Build history of the part. All positions in model axes, mm. A direction names the side the tool comes from. Round coordinates to 2 decimals unless told otherwise and drop trailing zeros. Order: outer loops, then holes, each group sorted by start corner. A loop starts at its lowest first (then second) coordinate and runs counter-clockwise, first axis right, second up. Notation, with made-up numbers: M 23,31 L 34,31 A17 ccw 34,35 Z; hole C -22,18.25 d3. An arc over 180 degrees is marked long. One line per question, with ' | ' between items. Start each with the question number.
from build123d import *

# Parameters (mm, degrees)
SM_BASE_FLANGE_1_DEPTH = 20
HOLE_WIZARD_M51_D      = 5.2
HOLE_WIZARD_M51_DEPTH  = 10
HOLE_WIZARD_M51_TIP    = 1.562237609


# Sheet-metal steps are written as plain solids
with BuildPart() as part:
    # Sketch 1 → Базовая кромка1 (new body)
    with BuildSketch(Plane(origin=(0, 0, 0), x_dir=(0, 0, -1), z_dir=(1, 0, 0))):
        with BuildLine():
            Line((0, 0), (0, 20))
            ThreePointArc((0, 20), (2.928932188, 27.071067812), (10, 30))
            Line((10, 30), (48.1, 30))
            ThreePointArc((48.1, 30), (55.171067812, 27.071067812), (58.1, 20))
            Line((58.1, 20), (58.1, 0))
            Line((58.1, 0), (68.1, 0))
            Line((68.1, 0), (68.1, 20))
            ThreePointArc((68.1, 20), (62.242135624, 34.142135624), (48.1, 40))
            Line((48.1, 40), (10, 40))
            ThreePointArc((10, 40), (-4.142135624, 34.142135624), (-10, 20))
            Line((-10, 20), (-10, 0))
            Line((-10, 0), (0, 0))
        make_face()
    extrude(amount=SM_BASE_FLANGE_1_DEPTH)

    # Сверло под метчик  спиральное M51
    with Locations(Plane(origin=(0, 0, 0), x_dir=(-1, 0, 0), z_dir=(0, -1, 0))):
        with Locations((-10, 63.1), (-10, -5)):
            Hole(HOLE_WIZARD_M51_D / 2, depth=HOLE_WIZARD_M51_DEPTH)
            with Locations((0, 0, -(HOLE_WIZARD_M51_DEPTH + HOLE_WIZARD_M51_TIP / 2))):  # 118° drill point
                Cone(0, HOLE_WIZARD_M51_D / 2, HOLE_WIZARD_M51_TIP, mode=Mode.SUBTRACT)


solid = part.part
Item 1: Tool access for faces 1 (the face through (9.86, 33.986, -62.397)), 2 (the face through (10, 30, -29)), 3 (the face through (9.662, 5.07, -65.678)): list every direction of +Z, -Z, +X, -X, +Y, -Y with a clear straight run to the whole face (end or side of a thin tool).
Item 2: Flat gauge pins, fed straight in: pin 1 (10 mm diameter, centred on x = 3, y = 30.5, fed in from +Z); pin 2 (4.5 mm diameter, centred on x = 10, z = 5, fed in from +Y); pin 3 (3 mm diameter, centred on x = 6, y = 34, fed in from -Z). Where does each tip first touch, or does it go through?
Item 3: Cut at B-B on y = 17.5. Write the cut outline in (x, z), then the cut area to 3 significant figures.
Item 4: Cut at D-D on z = -22.5. Write the cut outline in (x, y).
Item 5: Wall check: line 1 along Z through (x, y) = (9.75, 4); line 2 along Z through (x, y) = (15, 17.5); line 3 along Y through (x, z) = (3.75, -18). Give the ranges that are in metal, low to high. Write a range as [from, to].
Item 6: Cut at A-A on y = 4. Write the cut outline in (x, z), then the cut area to 3 significant figures.
Item 7: Two-plate mould, pull along Z, no slides. Class faces 4 (the face through (9.86, 34.297, 3.986)), 5 (the face through (9.86, 26.99, -2.85)), 6 (the face through (10, 40, -29)): +Z half, -Z half, draft (parallel to the pull), parting line (faces both ways), or undercut.
Item 8: Cut at C-C on x = 5.25. Write the cut outline in (y, z), then the cut area to 3 significant figures.
Results found:
1) face 1: -Z, +X, -X, +Y | face 2: +X, -X, -Y | face 3: -Y
2) pin 1: stops at z = 9.23 | pin 2: stops at y = 35.41 | pin 3: stops at z = -63.71
3) outline: M 0,-68.1 L 20,-68.1 L 20,-58.1 L 0,-58.1 Z; M 0,0 L 20,0 L 20,10 L 0,10 Z | area: 400 mm^2
4) outline: M 0,30 L 20,30 L 20,40 L 0,40 Z
5) line 1: z = [-68.1, -65.69], [-60.51, -58.1], [0, 2.41], [7.59, 10] | line 2: z = [-68.1, -58.1], [0, 10] | line 3: y = [30, 40]
6) outline: M 0,-68.1 L 20,-68.1 L 20,-58.1 L 0,-58.1 Z; M 0,0 L 20,0 L 20,10 L 0,10 Z; hole C 10,-63.1 d5.2; hole C 10,5 d5.2 | area: 358 mm^2
7) face 4: +Z half | face 5: undercut | face 6: draft
8) outline: M 0,-68.1 L 20,-68.1 A20 ccw 40,-48.1 L 40,-10 A20 ccw 20,10 L 0,10 L 0,0 L 20,0 A10 cw 30,-10 L 30,-48.1 A10 cw 20,-58.1 L 0,-58.1 Z | area: 1,250 mm^2
